Check sheet for the modelled part. Datum: model origin and axes. Units: mm. Face numbers are marked on the shaded views. A direction names the side the tool comes from. Round coordinates to 2 decimals unless told otherwise and drop trailing zeros. Write each loop counter-clockwise with the first axis right and the second up, starting at its lowest first coordinate (ties: lowest second). Pieces come first, ordered by that corner, then holes. Notation, with made-up numbers: (62, 39.5) -> (117, 39.5) arc R17 ccw to (117, 66.5) -> close; hole circle Ø9 at (-36.5, 80.5). An arc over 180 degrees is marked (long way). One line per item, written item: value.
from build123d import *

# Parameters (mm, degrees)
F0_W          = 50
F0_H          = 50
F1_DEPTH      = 50
F2_W          = 10
F2_H          = 40
F3_DEPTH      = 40
F4_R          = 10
F5_SIZE       = 20
F7_ANGLE_BACK = 90
F7_ANGLE      = 180
F10_DEPTH     = 10


with BuildPart() as f1:
    # F0 (on Front) → F1 (new body)
    with BuildSketch(Plane.XZ):
        with Locations((25, 25)):
            Rectangle(F0_W, F0_H)
    extrude(amount=F1_DEPTH)

    # F2 (on face) → F3 (cut)
    with BuildSketch(Plane.XY.offset(50)):
        with Locations((39, -30)):
            Rectangle(F2_W, F2_H)
    extrude(amount=-F3_DEPTH, mode=Mode.SUBTRACT)

    # F4
    f4_edges = [f1.edges().sort_by_distance(p)[0] for p in [
        (39, -10, 10),
    ]]
    fillet(f4_edges, radius=F4_R)

    # F5
    f5_edges = [f1.edges().sort_by_distance(p)[0] for p in [
        (47, -50, 50),
    ]]
    chamfer(f5_edges, length=F5_SIZE)

    # F6 (on face) → F7 (revolve, cut)
    with BuildSketch(Plane.XZ.offset(50), mode=Mode.PRIVATE) as f7_sk:
        Polygon((25, 20), (0, 50), (0, 0), (25, 0), align=None)
    revolve(f7_sk.sketch.rotate(Axis((0, -50, 25), (0, 0, -1)), -F7_ANGLE_BACK), axis=Axis((0, -50, 25), (0, 0, -1)), revolution_arc=F7_ANGLE, mode=Mode.SUBTRACT)

    # F9 (on face) → F10 (cut)
    with BuildSketch(Plane.XY.offset(50)):
        with BuildLine():
            ThreePointArc((0, -34.5079771981), (10.6066017178, -38.9013754803), (15, -49.5079771981))
            ThreePointArc((15, -49.5079771981), (14.9979819343, -49.7540217013), (14.9919282803, -50))
            Line((14.9919282803, -50), (25, -50))
            Line((25, -50), (25, -35))
            Line((25, -35), (15, -25))
            Line((15, -25), (0, -25))
            Line((0, -25), (0, -34.5079771981))
        make_face()
    extrude(amount=-F10_DEPTH, mode=Mode.SUBTRACT)


solid = f1.part
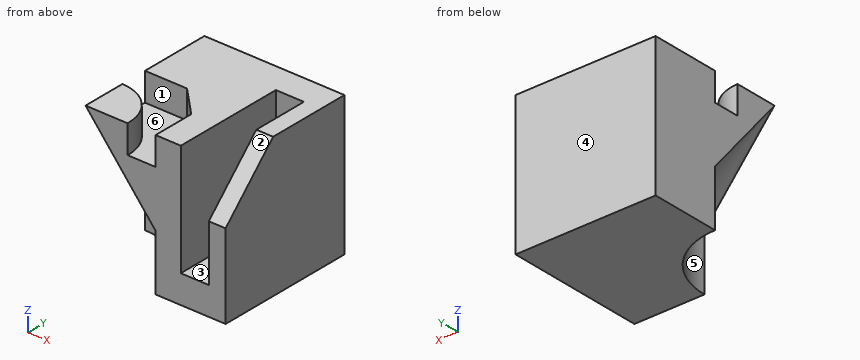
Item 1: Material ranges on line 1 along X through (y, z) = (-18, 36); line 2 along Y through (x, z) = (15, 10); line 3 along X through (y, z) = (-42.5, 24.5), recorded low to high.
Result set:
line 1: 0 to 34, 44 to 50
line 2: -30 to 0
line 3: 19.88 to 34, 44 to 50
Item 2: Sectioned sample at A-A (z = 44). Enter the section's corners in (x, y), then the cut area to 3 significant figures.
Result set:
outline: (0, -45) arc R5 cw to (5, -50) -> (14.99, -50) arc R15 ccw to (0, -34.51) -> close; (0, -25) -> (15, -25) -> (25, -35) -> (25, -50) -> (34, -50) -> (34, -10) -> (44, -10) -> (44, -36) -> (50, -36) -> (50, 0) -> (0, 0) -> close
area: 1,610 mm^2
Item 3: Depth check by flat-ended pin: pin 1 (5 mm diameter, centred on x = 37.5, y = -30.5, fed in from +Z). Enter the tip coordinate at first touch or a pass-through.
Result set:
pin 1: z = 10
Item 4: Sectioned sample at C-C (y = -19). Enter the section's corners in (x, z), then the cut area to 3 significant figures.
Result set:
outline: (0, 0) -> (50, 0) -> (50, 50) -> (44, 50) -> (44, 10.05) -> (34, 10.05) -> (34, 50) -> (0, 50) -> close
area: 2,100 mm^2
Item 5: Sectioned sample at B-B (x = 39.5). Enter the section's corners in (y, z).
Result set:
outline: (-50, 0) -> (0, 0) -> (0, 50) -> (-10, 50) -> (-10, 20) arc R10 cw to (-20, 10) -> (-50, 10) -> close
Item 6: Tool access check on the marked faces 1, 2 and 3. Record the directions out of +Z, -Z, +X, -X, +Y, -Y that give a thin tool (end or side, any length) a straight path to the whole face; none if there is none.
Result set:
face 1: +Z, -X
face 2: +Z, +X, -Y
face 3: +Z, -Y
Item 7: Release check for a two-part mould opening along X. For the marked faces 4, 5 and 6 record: pulls with the +X half, pulls with the -X half, needs draft (parallel to the pull), parting line crosses it, or undercut.
Result set:
face 4: needs draft
face 5: pulls with the -X half
face 6: undercut
Item 8: Sectioned sample at D-D (z = 31). Enter the section's corners in (x, y), then the cut area to 3 significant figures.
Result set:
outline: (0, -34.17) arc R15.83 cw to (15.83, -50) -> (34, -50) -> (34, -10) -> (44, -10) -> (44, -49) -> (50, -49) -> (50, 0) -> (0, 0) -> close
area: 1,900 mm^2
